```python
from build123d import *

# Parameters (mm, degrees)
F0_W           = 60
F0_H           = 40
F1_DEPTH       = 2
F2_W           = 60
F2_H           = 40
F2_W_2         = 46
F2_H_2         = 26
F3_DEPTH       = 4
F4_W           = 53
F4_H           = 33
F4_W_2         = 46
F4_H_2         = 26
F5_DEPTH       = 25
F6_R           = 5
F7_R           = 2
F9_DEPTH       = 36.501
F11_DEPTH      = 8
F11_DEPTH_BACK = 8


with BuildPart() as f1:
    # F0 (on Top) → F1 (new body)
    with BuildSketch(Plane.XY):
        Rectangle(F0_W, F0_H)
    extrude(amount=F1_DEPTH)

    # F2 (on face) → F3 (join)
    with BuildSketch(Plane.XY.offset(2)):
        Rectangle(F2_W, F2_H)
        Rectangle(F2_W_2, F2_H_2, mode=Mode.SUBTRACT)
    extrude(amount=F3_DEPTH)

    # F4 (on face) → F5 (join)
    with BuildSketch(Plane.XY.offset(6)):
        Rectangle(F4_W, F4_H)
        Rectangle(F4_W_2, F4_H_2, mode=Mode.SUBTRACT)
    extrude(amount=F5_DEPTH)

    # F6
    f6_edges = [f1.edges().sort_by_distance(p)[0] for p in [
        (-26.5, -16.5, 18.5),
        (26.5, -16.5, 18.5),
        (-26.5, 16.5, 18.5),
        (-30, -20, 3),
        (30, -20, 3),
        (-30, 20, 3),
        (30, 20, 3),
        (26.5, 16.5, 18.5),
    ]]
    fillet(f6_edges, radius=F6_R)

    # F7
    f7_edges = [f1.edges().sort_by_distance(p)[0] for p in [
        (0, 16.5, 31),
        (0, 20, 0),
        (23, -13, 16.5),
        (-23, -13, 16.5),
        (23, 13, 16.5),
        (23, 0, 2),
        (0, 13, 2),
        (0, -13, 2),
        (-23, 0, 2),
    ]]
    fillet(f7_edges, radius=F7_R)

    # F8 (on face) → F9 (cut, through all)
    with BuildSketch(Plane.XZ.offset(16.5)):
        Polygon((10, 21), (-10, 21), (-10, 9), (-8, 9), (-8, 19), (8, 19), (8, 9), (10, 9), align=None)
    extrude(amount=-F9_DEPTH, mode=Mode.SUBTRACT)

    # F10 (on Right) → F11 (join, two sides)
    with BuildSketch(Plane.YZ) as f11_sk:
        Polygon((-18.5, 17), (-16.5, 14), (-16.5, 19), align=None)
        Polygon((16.5, 19), (16.5, 14), (18.5, 17), align=None)
    extrude(amount=F11_DEPTH)
    extrude(f11_sk.sketch, amount=-F11_DEPTH_BACK)


solid = f1.part
```
Source: CAD feature listing. Evaluate the final solid. Frame: model axes, mm. A direction names the side the tool comes from. Round coordinates to 2 decimals unless told otherwise and drop trailing zeros. Loops run counter-clockwise (first coordinate to the right, second up) from the corner with the lowest first, then second, coordinate; pieces in that order, holes last. Notation, with made-up numbers: M -30,-36.75 L 15,-36.75 A24 cw 15,-3.75 Z; hole C -16.75,-35 d11. An arc over 180 degrees is marked long. Use a Markdown table: item, result. Add a question column.
1. Section query B-B on x = 3. Give the number of separate pieces and of enclosed holes in the cut face, then the cut area to 3 significant figures.
2. Contact query for flat-ended pins moving along their axis: P1, Ø6, axis at y = -15.5, z = 12, coming from the +X side; P2, Ø12, axis at y = -3.5, z = 24, coming from the +X side; P3, Ø6.5, axis at y = -1, z = 13, coming from the -X side. Output: stop coordinate, or through.
3. Reachability of faces 5 (the flat face through (0, 14, 31)), 6 (the flat face through (23, 0, 17)), 7 (the flat face through (8, -15, 14)) from +Z, -Z, +X, -X, +Y, -Y: full face, straight path, thin tool, end or side. Return the list, or none.
4. Section query A-A on z = 24.5. Return the cut outline in (x, y).
5. Line query: line 1 (X direction, y = -0.5, z = 25); line 2 (Y direction, x = 3, z = 5); line 3 (Y direction, x = 3.5, z = 22). Output: solid intervals per line, ascending.
6. Section query D-D on y = -3. Return the cut outline in (x, z), then the cut area to 3 significant figures.
7. Section query C-C on z = 20. Return the cut outline in (x, y).
8. Mould query, pull axis X, two halves, no side actions, for faces 1 (the flat face through (0.1, -17.5, 18)), 2 (the cylindrical face through (-28, 19, 4)), 3 (the cylindrical face through (25.07, 15, 17.66)), 4 (the flat face through (-8, 15, 14)). Classes: pulls with the +X half, pulls with the -X half, needs draft (parallel to the pull), parting line crosses it, or undercut.
Reported:
| question | item | result |
|---|---|---|
| 1 | separate pieces | 3 |
| 1 | enclosed holes | 0 |
| 1 | area | 305 mm² |
| 2 | P1 | stops at x = 26.4 |
| 2 | P2 | stops at x = 26.5 |
| 2 | P3 | stops at x = -26.5 |
| 3 | face 5 | +Z, +X, -X, +Y, -Y |
| 3 | face 6 | +Z |
| 3 | face 7 | +Y, -Y |
| 4 | outline | M -26.5,-11.5 A5 ccw -21.5,-16.5 L 21.5,-16.5 A5 ccw 26.5,-11.5 L 26.5,11.5 A5 ccw 21.5,16.5 L -21.5,16.5 A5 ccw -26.5,11.5 Z; hole M -23,-11 A2 ccw -21,-13 L 21,-13 A2 ccw 23,-11 L 23,11 A2 ccw 21,13 L -23,13 Z |
| 5 | line 1 | x = -26.5 to -23, 23 to 26.5 |
| 5 | line 2 | y = -20 to -13, 13 to 20 |
| 5 | line 3 | y = -16.5 to -13, 13 to 16.5 |
| 6 | outline | M -30,2 A2 ccw -28,0 L 28,0 A2 ccw 30,2 L 30,6 L 26.5,6 L 26.5,29 A2 ccw 24.5,31 L 23,31 L 23,4 A2 cw 21,2 L -21,2 A2 cw -23,4 L -23,31 L -24.5,31 A2 ccw -26.5,29 L -26.5,6 L -30,6 Z |
| 6 | area | 349 mm² |
| 7 | outline | M -26.5,-11.5 A5 ccw -21.5,-16.5 L -10,-16.5 L -10,-13 L -21,-13 A2 cw -23,-11 L -23,13 L -10,13 L -10,16.5 L -21.5,16.5 A5 ccw -26.5,11.5 Z; M 10,-16.5 L 21.5,-16.5 A5 ccw 26.5,-11.5 L 26.5,11.5 A5 ccw 21.5,16.5 L 10,16.5 L 10,13 L 21,13 A2 cw 23,11 L 23,-11 A2 cw 21,-13 L 10,-13 Z |
| 8 | face 1 | needs draft |
| 8 | face 2 | pulls with the -X half |
| 8 | face 3 | pulls with the +X half |
| 8 | face 4 | undercut |
